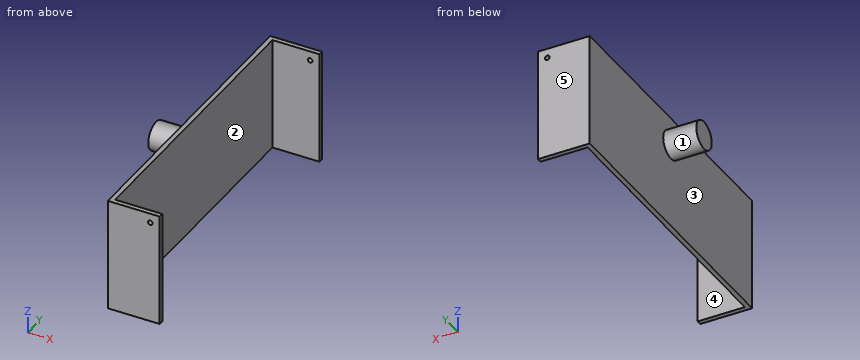
from build123d import *

# Parameters (mm, degrees)
BOSS_EXTRUDE1_DEPTH = 120
SKETCH2_R           = 15
BOSS_EXTRUDE2_DEPTH = 35
SKETCH3_R           = 2.5
CUT_EXTRUDE1_DEPTH  = 320


with BuildPart() as part:
    # Sketch1 → Boss-Extrude1 (new body)
    with BuildSketch(Plane.XY):
        Polygon((-5, 5), (50, 5), (50, 0), (0, 0), (0, -305), (50, -305), (50, -310), (-5, -310), align=None)
    extrude(amount=BOSS_EXTRUDE1_DEPTH)

    # Sketch2 → Boss-Extrude2 (add)
    with BuildSketch(Plane.ZY.offset(5)):
        with Locations(Location((90, -152.5, 0), (0, 0, 90))):
            Circle(SKETCH2_R)
    extrude(amount=BOSS_EXTRUDE2_DEPTH)

    # Sketch3 → Cut-Extrude1 (cut)
    with BuildSketch(Plane.XZ.offset(310)):
        with Locations(Location((40, 110, 0), (0, 0, 270))):
            Circle(SKETCH3_R)
    extrude(amount=-CUT_EXTRUDE1_DEPTH, mode=Mode.SUBTRACT)


solid = part.part
Model file for the job. Use its own axes, mm. Face numbers are marked on the shaded views. A direction names the side the tool comes from. Round coordinates to 2 decimals unless told otherwise and drop trailing zeros. Order: outer loops, then holes, each group sorted by start corner. A loop starts at its lowest first (then second) coordinate and runs counter-clockwise, first axis right, second up. Notation, with made-up numbers: M 67,4 L 99,4 A34 cw 99,35 Z; hole C 8.25,-25.75 d1. An arc over 180 degrees is marked long. Write each question's results on one line, items separated by ' | '. Start each with the question number.
(1) Saw through at D-D, the plane z = 65.5. Give the cut face in (x, y).
(2) Probe probe 1 along X at (y, z) = (-306.5, 110); probe 2 along Y at (x, z) = (40, 26); probe 3 along X at (y, z) = (-263, 35). List the from-to ranges inside material, lowest first. Write a range as from..to.
(3) Drop flat-ended pins along their axis: pin 1 (2 mm diameter, centred on y = -219.5, z = 79.5, fed in from -X); pin 2 (4 mm diameter, centred on x = 40, z = 110, fed in from -Y); pin 3 (1 mm diameter, centred on x = -23, y = -147, fed in from +Z); pin 4 (1.5 mm diameter, centred on y = -210, z = 87, fed in from +X). Give the stop position or say it passes through.
(4) Saw through at B-B, the plane z = 90. Give the cut face in (x, y), then the cut area to 4 significant figures.
(5) Which spindle directions (+Z, -Z, +X, -X, +Y, -Y) get a long thin tool onto all of the face, cutting with end or side? Do the marked faces 4 and 5. Say none if no direction does.
(6) Saw through at A-A, the plane x = 29. Give the cut face in (y, z), then the cut area to 3 significant figures.
(7) Two-plate mould, pull along Y, no slides. Class the marked faces 1, 2 and 3: pulls with the +Y half, pulls with the -Y half, needs draft (parallel to the pull), parting line crosses it, or undercut.
(8) Saw through at C-C, the plane y = -152.5. Give the cut face in (x, z).
Established:
1) outline: M -5,-310 L 50,-310 L 50,-305 L 0,-305 L 0,0 L 50,0 L 50,5 L -5,5 Z
2) probe 1: x = -5..37.5, 42.5..50 | probe 2: y = -310..-305, 0..5 | probe 3: x = -5..0
3) pin 1: stops at x = -5 | pin 2: passes through | pin 3: stops at z = 104.14 | pin 4: stops at x = 0
4) outline: M -40,-167.5 L -5,-167.5 L -5,-310 L 50,-310 L 50,-305 L 0,-305 L 0,0 L 50,0 L 50,5 L -5,5 L -5,-137.5 L -40,-137.5 Z | area: 3,125 mm^2
5) face 4: +Z, -Z, +X | face 5: +Z, -Z, +X, -X, +Y
6) outline: M -310,0 L -305,0 L -305,120 L -310,120 Z; M 0,0 L 5,0 L 5,120 L 0,120 Z | area: 1,200 mm^2
7) face 1: parting line crosses it | face 2: undercut | face 3: needs draft
8) outline: M -40,75 L -5,75 L -5,0 L 0,0 L 0,120 L -5,120 L -5,105 L -40,105 Z
